Geometry: final body of the model. Coordinates: model frame, mm. A direction names the side the tool comes from. Give positions to 0.01 mm unless a question says otherwise; leave off trailing zeros. Order: outer loops, then holes, each group sorted by start corner. A loop starts at its lowest first (then second) coordinate and runs counter-clockwise, first axis right, second up. Notation, with made-up numbers: (-11, 55.5) - (33, 55.5) arc R18 ccw to (33, 60.5) - close; hole circle Ø5 at (-1.75, -14.5). An arc over 180 degrees is marked (long way). One line per question, with ' | ' between items. Start each with the question number.
from build123d import *

# Parameters (mm, degrees)
SKETCH_1_R          = 1.5
EXTRUDE_1_DEPTH     = 3
CUT_EXTRUDE_1_DEPTH = 22.104738804


with BuildPart() as part:
    # 草图1 → 凸台-拉伸1 (new body)
    with BuildSketch(Plane(origin=(0, 0, 0), x_dir=(1, 0, 0), z_dir=(0, 1, 0))):
        with BuildLine():
            Line((15.9, 4.5), (-15.9, 4.5))
            ThreePointArc((-15.9, 4.5), (-20.4, 0), (-15.9, -4.5))
            Line((-15.9, -4.5), (15.9, -4.5))
            ThreePointArc((15.9, -4.5), (20.4, 0), (15.9, 4.5))
        make_face()
        with Locations(Location((-15.9, 0, 0), (0, 0, 270))):
            Circle(SKETCH_1_R, mode=Mode.SUBTRACT)
        with Locations(Location((15.9, 0, 0), (0, 0, 270))):
            Circle(SKETCH_1_R, mode=Mode.SUBTRACT)
    extrude(amount=EXTRUDE_1_DEPTH)

    # 草图2 → 切除-拉伸1 (cut, through all)
    with BuildSketch(Plane(origin=(0, 3, 0), x_dir=(1, 0, 0), z_dir=(0, 1, 0))):
        with BuildLine():
            Line((-10, 2.5), (10, 2.5))
            ThreePointArc((10, 2.5), (12.5, 0), (10, -2.5))
            Line((10, -2.5), (-10, -2.5))
            ThreePointArc((-10, -2.5), (-12.5, 0), (-10, 2.5))
        make_face()
    extrude(amount=-CUT_EXTRUDE_1_DEPTH, mode=Mode.SUBTRACT)


solid = part.part
(1) Access query for faces 1 (the flat face through (0, 2, -2.5)), 2 (the flat face through (0, 0, 3)). Directions: +Z, -Z, +X, -X, +Y, -Y. A direction counts if a zero-diameter tool reaches every point of the face in a straight line with its end or side. Return the directions, or none.
(2) Cut plane C-C, the plane y = 1.65. Return the cut outline in (x, z).
(3) Contact query for a flat-ended pin moving along its axis: P1, Ø1.8, axis at x = -15.9, z = 0, coming from the -Y side. Output: stop coordinate, or through.
(4) Material intervals for line 1 along X through (y, z) = (0.65, 0); line 2 along X through (y, z) = (0.5, 1); line 3 along Z through (x, y) = (4, 2.75), sorted ascending. Write a range as from..to.
(5) Cut plane A-A, the plane z = 0. Return the cut outline in (x, y).
(6) Cut plane D-D, the plane z = 3.5. Return the cut outline in (x, y).
(7) Pull-direction query (Z, two-part tool) for faces 3 (the cylindrical face through (20.4, 1.5, 0.1)), 4 (the flat face through (0, 3, 3)), 5 (the cylindrical face through (-12.5, 1.5, 0.1)); classes: +Z half, -Z half, draft (parallel to the pull), parting line (faces both ways), or undercut.
(8) Cut plane B-B, the plane x = -1.5. Return the cut outline in (y, z), plus the area to 3 significant figures.
Results are:
1) face 1: +Y, -Y | face 2: +Z, -Z, +X, -X, -Y
2) outline: (-15.9, -4.5) - (15.9, -4.5) arc R4.5 ccw to (15.9, 4.5) - (-15.9, 4.5) arc R4.5 ccw to start; hole circle Ø3 at (-15.9, 0); hole (-10, -2.5) - (10, -2.5) arc R2.5 ccw to (10, 2.5) - (-10, 2.5) arc R2.5 ccw to start; hole circle Ø3 at (15.9, 0)
3) P1: through
4) line 1: -20.4..-17.4, -14.4..-12.5, 12.5..14.4, 17.4..20.4 | line 2: -20.29..-17.02, -14.78..-12.29, 12.29..14.78, 17.02..20.29 | line 3: -4.5..-2.5, 2.5..4.5
5) outline: (-20.4, 0) - (-17.4, 0) - (-17.4, 3) - (-20.4, 3) - close; (-14.4, 0) - (-12.5, 0) - (-12.5, 3) - (-14.4, 3) - close; (12.5, 0) - (14.4, 0) - (14.4, 3) - (12.5, 3) - close; (17.4, 0) - (20.4, 0) - (20.4, 3) - (17.4, 3) - close
6) outline: (-18.73, 0) - (18.73, 0) - (18.73, 3) - (-18.73, 3) - close
7) face 3: parting line | face 4: draft | face 5: undercut
8) outline: (0, -4.5) - (3, -4.5) - (3, -2.5) - (0, -2.5) - close; (0, 2.5) - (3, 2.5) - (3, 4.5) - (0, 4.5) - close | area: 12.0 mm2
